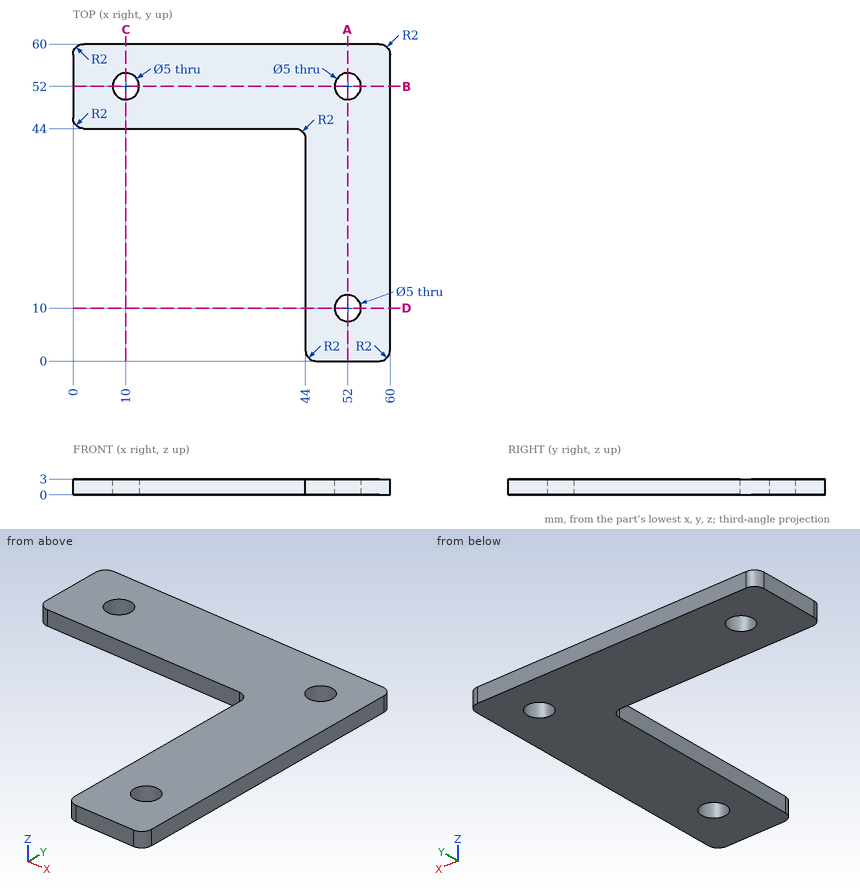
Design review of the part shown in the three views and the two pictorial views. Dimensions are in mm from the part's minimum x, y and z. Round coordinates to 2 decimals unless told otherwise and drop trailing zeros. Loops run counter-clockwise (first coordinate to the right, second up) from the corner with the lowest first, then second, coordinate; pieces in that order, holes last. Notation, with made-up numbers: (48.25, 15.5) -> (68.25, 15.5) arc R19 ccw to (68.25, 47.5) -> close; hole circle Ø8 at (32, 78.5). An arc over 180 degrees is marked (long way). Use one line per item in the form item = value. Start each with the question number.
Q1. For pin 1 Ø0.9 at (y, z) = (14, 1.5) entering from -X, flat-tipped, find the tip position at first contact; note if it passes through.
Q2. Wall thickness on line 1 along Y through (x, z) = (52, 1.3); line 2 along Y through (x, z) = (10, 1.85); line 3 along X through (y, z) = (24.5, 2.75): over which ranges is each line inside the solid? List them lowest first. Write a range as [from, to].
Q3. We need section C-C on x = 10. Give the boundary of the cut face in (y, z), then the cut area to 3 significant figures.
Q4. We need section A-A on x = 52. Give the boundary of the cut face in (y, z).
Calculated:
q1.pin_1 = 44
q2.line_1 = [0, 7.5], [12.5, 49.5], [54.5, 60]
q2.line_2 = [44, 49.5], [54.5, 60]
q2.line_3 = [44, 60]
q3.outline = (44, 0) -> (49.5, 0) -> (49.5, 3) -> (44, 3) -> close; (54.5, 0) -> (60, 0) -> (60, 3) -> (54.5, 3) -> close
q3.area = 33.0 mm²
q4.outline = (0, 0) -> (7.5, 0) -> (7.5, 3) -> (0, 3) -> close; (12.5, 0) -> (49.5, 0) -> (49.5, 3) -> (12.5, 3) -> close; (54.5, 0) -> (60, 0) -> (60, 3) -> (54.5, 3) -> close
